from build123d import *

# Parameters (mm, degrees)
F1_DEPTH = 5
F3_D     = 5.5
F5_D     = 6.7564
F7_D     = 4


with BuildPart() as f1:
    # F0 (on Top) → F1 (new body)
    with BuildSketch(Plane.XY):
        Polygon((0, 88), (0, 0), (89, 0), (89, 77), align=None)
    extrude(amount=-F1_DEPTH)

    # F3 (through all)
    with Locations(Plane.XY):
        with Locations((5, 5), (5, 81.75), (83.5, 71.5)):
            Hole(F3_D / 2)

    # F5 (through all)
    with Locations(Plane.XY):
        with Locations((44.5, 41)):
            Hole(F5_D / 2)

    # F7 (through all)
    with Locations(Plane.XY):
        with Locations((44.5, 55), (44.5, 27)):
            Hole(F7_D / 2)


solid = f1.part
Model file for the job. Use its own axes, mm. Give positions to 0.01 mm unless a question says otherwise; leave off trailing zeros. Loops run counter-clockwise (first coordinate to the right, second up) from the corner with the lowest first, then second, coordinate; pieces in that order, holes last. Notation, with made-up numbers: (68.5, 69) -> (92.5, 69) arc R24 cw to (92.5, 102) -> close; hole circle Ø10 at (54.25, -9). An arc over 180 degrees is marked (long way). Use a Markdown table: item, result. Add a question column.
(1) Drop flat-ended pins along their axis: pin 1 Ø5.5 at (x, y) = (44.5, 41) entering from -Z; pin 2 Ø1.5 at (x, z) = (40.5, -3) entering from +Y. Give the stop position or say it passes through.
(2) Mould opens along Y. For faces 1 (the flat face through (44, 45, 0)), 2 (the cylindrical face through (44.934, 25.048, -2.535)), 3 (the flat face through (45.123, 82.423, -2.465)), 4 (the flat face through (44, 0, -2)) say: +Y half, -Y half, draft (parallel to the pull), parting line (faces both ways), or undercut.
(3) Slice it at B-B on x = 44.5. List the corners of the cut face in (y, z).
(4) Wall check: line 1 along Y through (x, z) = (44.5, -3.3); line 2 along Y through (x, z) = (4, -0.95); line 3 along Y through (x, z) = (82, -3.5). Give the ranges that are in metal, low to high.
(5) Slice it at A-A on y = 55. List the corners of the cut face in (x, z).
(6) Slice it at C-C on z = -0.85. List the corners of the cut face in (x, y), and give its area (3 significant figures).
(7) Slice it at D-D on x = 83.5. List the corners of the cut face in (y, z).
Filled sheet:
| question | item | result |
|---|---|---|
| 1 | pin 1 | through |
| 1 | pin 2 | y = 83.09 |
| 2 | face 1 | draft |
| 2 | face 2 | undercut |
| 2 | face 3 | +Y half |
| 2 | face 4 | -Y half |
| 3 | outline | (0, -5) -> (25, -5) -> (25, 0) -> (0, 0) -> close; (29, -5) -> (37.62, -5) -> (37.62, 0) -> (29, 0) -> close; (44.38, -5) -> (53, -5) -> (53, 0) -> (44.38, 0) -> close; (57, -5) -> (82.5, -5) -> (82.5, 0) -> (57, 0) -> close |
| 4 | line 1 | 0 to 25, 29 to 37.62, 44.38 to 53, 57 to 82.5 |
| 4 | line 2 | 0 to 2.44, 7.56 to 79.19, 84.31 to 87.51 |
| 4 | line 3 | 0 to 69.2, 73.8 to 77.87 |
| 5 | outline | (0, -5) -> (42.5, -5) -> (42.5, 0) -> (0, 0) -> close; (46.5, -5) -> (89, -5) -> (89, 0) -> (46.5, 0) -> close |
| 6 | outline | (0, 0) -> (89, 0) -> (89, 77) -> (0, 88) -> close; hole circle Ø5.5 at (5, 5); hole circle Ø5.5 at (5, 81.75); hole circle Ø6.76 at (44.5, 41); hole circle Ø4 at (44.5, 27); hole circle Ø4 at (44.5, 55); hole circle Ø5.5 at (83.5, 71.5) |
| 6 | area | 7,210 mm2 |
| 7 | outline | (0, -5) -> (68.75, -5) -> (68.75, 0) -> (0, 0) -> close; (74.25, -5) -> (77.68, -5) -> (77.68, 0) -> (74.25, 0) -> close |
